Input: part model. Units: mm. Frame: model coordinates. A direction names the side the tool comes from. Give positions to 0.01 mm unless a question says otherwise; leave off trailing zeros. Loops run counter-clockwise (first coordinate to the right, second up) from the corner with the lowest first, then second, coordinate; pieces in that order, holes last. Notation, with made-up numbers: M -18.5,-36.75 L 31.5,-36.75 A28 ccw 31.5,-5.75 Z; hole C 45,79 d10. An arc over 180 degrees is marked long. Use a Markdown table: item, result. Add a question column.
from build123d import *

# Parameters (mm, degrees)
F1_DEPTH  = 25.4
F3_W      = 25.4
F3_H      = 25.4
F4_DEPTH  = 25.401
F5_R      = 12.7
F6_DEPTH  = 38.1
F8_DEPTH  = 12.701
F10_DEPTH = 38.101
F11_R     = 6.35
F12_DEPTH = 38.101
F14_DEPTH = 38.101


with BuildPart() as f1:
    # F0 (on Front) → F1 (new body)
    with BuildSketch(Plane.XZ):
        Polygon((25.4, 38.1), (0, 38.1), (0, 0), (82.55, 0), (82.55, 12.7), (25.4, 12.7), align=None)
    extrude(amount=F1_DEPTH)

    # F3 (on Front) → F4 (cut, through all)
    with BuildSketch(Plane.XZ):
        with Locations((12.7, 25.4)):
            Rectangle(F3_W, F3_H)
    extrude(amount=F4_DEPTH, mode=Mode.SUBTRACT)

    # F5 (on Top) → F6 (join)
    with BuildSketch(Plane.XY):
        with Locations((12.7, -12.7)):
            Circle(F5_R)
    extrude(amount=F6_DEPTH)

    # F8 (cut, through all): faces of the model
    f8_faces = [f1.faces().sort_by_distance(p)[0] for p in [
        (2.8367728246, -2.8367728246, 12.7),
        (2.8367728246, -22.5632271754, 12.7),
    ]]
    extrude(f8_faces, amount=-F8_DEPTH, mode=Mode.SUBTRACT)

    # F9 (on Top) → F10 (cut, through all)
    with BuildSketch(Plane.XY):
        with BuildLine():
            ThreePointArc((70.9260618119, -18.9581619488), (74.7056921497, -16.792035404), (76.2, -12.7))
            ThreePointArc((76.2, -12.7), (74.3718130047, -8.2417820656), (69.9399347557, -6.3506369028))
            Line((69.9399347557, -6.3506369028), (69.7600652443, -6.3506369028))
            ThreePointArc((69.7600652443, -6.3506369028), (63.5180353707, -12.2217490892), (68.8073960441, -18.9638228735))
            Line((68.8073960441, -18.9638228735), (70.9260618119, -18.9581619488))
        make_face()
        with BuildLine():
            Line((69.7600652443, -6.3506369028), (69.9399347557, -6.3506369028))
            ThreePointArc((69.9399347557, -6.3506369028), (69.85, -6.35), (69.7600652443, -6.3506369028))
        make_face()
        with BuildLine():
            ThreePointArc((68.8073960441, -18.9638228735), (69.8669666894, -19.0499773331), (70.9260618119, -18.9581619488))
            Line((70.9260618119, -18.9581619488), (68.8073960441, -18.9638228735))
        make_face()
        with BuildLine():
            ThreePointArc((68.8073960441, -18.9638228735), (63.5180353707, -12.2217490892), (69.7600652443, -6.3506369028))
            Line((69.7600652443, -6.3506369028), (38.1899347557, -6.3506369028))
            ThreePointArc((38.1899347557, -6.3506369028), (42.6218130047, -8.2417820656), (44.45, -12.7))
            ThreePointArc((44.45, -12.7), (42.6764639727, -17.1020992158), (38.3465425178, -19.0452121152))
            Line((38.3465425178, -19.0452121152), (68.8073960441, -18.9638228735))
        make_face()
        with BuildLine():
            Line((38.0100652443, -6.3506369028), (38.1899347557, -6.3506369028))
            ThreePointArc((38.1899347557, -6.3506369028), (38.1, -6.35), (38.0100652443, -6.3506369028))
        make_face()
        with BuildLine():
            ThreePointArc((44.45, -12.7), (42.6218130047, -8.2417820656), (38.1899347557, -6.3506369028))
            Line((38.1899347557, -6.3506369028), (38.0100652443, -6.3506369028))
            ThreePointArc((38.0100652443, -6.3506369028), (31.7502965226, -12.6386342958), (37.8873686745, -19.0464389952))
            Line((37.8873686745, -19.0464389952), (38.3465425178, -19.0452121152))
            ThreePointArc((38.3465425178, -19.0452121152), (42.6764639727, -17.1020992158), (44.45, -12.7))
        make_face()
        with BuildLine():
            ThreePointArc((37.8873686745, -19.0464389952), (38.1169666894, -19.0499773331), (38.3465425178, -19.0452121152))
            Line((38.3465425178, -19.0452121152), (37.8873686745, -19.0464389952))
        make_face()
    extrude(amount=F10_DEPTH, mode=Mode.SUBTRACT)

    # F11 (on Top) → F12 (cut, through all)
    with BuildSketch(Plane.XY):
        with Locations((12.6997202718, -12.7842912701)):
            Circle(F11_R)
    extrude(amount=F12_DEPTH, mode=Mode.SUBTRACT)

    # F13 (on Top) → F14 (cut, through all)
    with BuildSketch(Plane.XY):
        with BuildLine():
            ThreePointArc((69.85, 0), (78.8302561211, -3.7197438789), (82.55, -12.7))
            Line((82.55, -12.7), (82.55, 0))
            Line((82.55, 0), (69.85, 0))
        make_face()
        with BuildLine():
            ThreePointArc((82.55, -12.7), (78.8302561211, -21.6802561211), (69.85, -25.4))
            Line((69.85, -25.4), (82.55, -25.4))
            Line((82.55, -25.4), (82.55, -12.7))
        make_face()
    extrude(amount=F14_DEPTH, mode=Mode.SUBTRACT)


solid = f1.part
1) Section query B-B, the plane y = -7.25. Return the cut outline in (x, z), and give its area (3 significant figures).
2) Section query C-C, the plane z = 10. Return the cut outline in (x, y).
3) Contact query for flat-ended pins moving along their axis: P1, Ø12, axis at y = -9, z = 11, coming from the +X side; P2, Ø1, axis at y = -8.5, z = 33, coming from the -X side; P3, Ø2, axis at x = 39.5, y = -8.5, coming from the -Z side; P4, Ø6, axis at x = 46.5, y = -4.5, coming from the +Z side. Output: stop coordinate, or through.
4) Pull-direction query (Y, two-part tool) for faces 1 (the flat face through (41, 0, 6)), 2 (the flat face through (54, -6.351, 6)), 3 (the flat face through (6.9, -9.7, 38.1)); classes: pulls with the +Y half, pulls with the -Y half, needs draft (parallel to the pull), parting line crosses it, or undercut.
5) Section query A-A, the plane x = 40.5. Return the cut outline in (y, z).
6) Section query D-D, the plane y = -1.75. Return the cut outline in (x, z).
7) Ray query, line 1 (Y direction, x = 43.5, z = 9.5); line 2 (X direction, y = -13.5, z = 2.5); line 3 (Z direction, x = 66.5, y = -20.25). Return the intervals inside material, ascending. Write a range as [from, to].
8) Reachability of faces 4 (the cylindrical face through (0.012, -13.258, 23.55)), 5 (the flat face through (31.5, -12.5, 0)) from +Z, -Z, +X, -X, +Y, -Y: full face, straight path, thin tool, end or side. Return the list, or none.
Entries:
| question | item | result |
|---|---|---|
| 1 | outline | M 1.23,0 L 9.59,0 L 9.59,38.1 L 1.23,38.1 Z; M 15.81,0 L 34.84,0 L 34.84,12.7 L 24.17,12.7 L 24.17,38.1 L 15.81,38.1 Z; M 73.11,0 L 81.32,0 L 81.32,12.7 L 73.11,12.7 Z |
| 1 | area | 877 mm² |
| 2 | outline | M 12.7,-25.4 L 69.85,-25.4 A12.7 ccw 69.85,0 L 12.7,0 A12.7 ccw Z; hole C 12.7,-12.78 d12.7; hole M 38.19,-6.35 A6.35 ccw long 38.35,-19.05 L 68.81,-18.96 A6.35 ccw long 69.76,-6.35 Z |
| 3 | P1 | stops at x = 82.55 |
| 3 | P2 | stops at x = 0.55 |
| 3 | P3 | passes through |
| 3 | P4 | stops at z = 12.7 |
| 4 | face 1 | pulls with the +Y half |
| 4 | face 2 | undercut |
| 4 | face 3 | needs draft |
| 5 | outline | M -25.4,0 L -19.04,0 L -19.04,12.7 L -25.4,12.7 Z; M -6.35,0 L 0,0 L 0,12.7 L -6.35,12.7 Z |
| 6 | outline | M 6.27,0 L 76.28,0 L 76.28,12.7 L 19.13,12.7 L 19.13,38.1 L 6.27,38.1 Z |
| 7 | line 1 | y = [-25.4, -19.03], [-6.35, 0] |
| 7 | line 2 | x = [0.03, 6.39], [19.01, 31.8], [76.15, 82.52] |
| 7 | line 3 | z = [0, 12.7] |
| 8 | face 4 | +Z |
| 8 | face 5 | -Z, +X, -X, +Y, -Y |
